Here's how the part is built. I have some questions about the finished solid (model axes, mm). A direction names the side the tool comes from. Round coordinates to 2 decimals unless told otherwise and drop trailing zeros. Write each loop counter-clockwise with the first axis right and the second up, starting at its lowest first coordinate (ties: lowest second). Pieces come first, ordered by that corner, then holes. Notation, with made-up numbers: M -13,-23 L 28,-23 A29 cw 28,16 Z; hole C 35,23 d5. An arc over 180 degrees is marked long. Use one line per item in the form item = value. Start each with the question number.
Q1. We'd pull the mould along X, two halves only. Please class faces 1 (the face through (-7, 12, 2)), 2 (the face through (-3.04, -11.29, -3.32)), 3 (the face through (-6.834, -8.007, -1.517)): +X half, -X half, draft (parallel to the pull), parting line (faces both ways), or undercut.
Q2. I need wall thicknesses on line 1 along X through (y, z) = (-11.4, 0); line 2 along Y through (x, z) = (-2.75, 6.5); line 3 along X through (y, z) = (6.5, 0). Which ranges of each line are inside material? Lowest first, please. Write a range as from..to.
Q3. I'm going to push flat-ended pins straight in: pin 1 Ø4.5 at (x, z) = (1.5, 2.5) entering from -Y; pin 2 Ø6 at (x, z) = (0.5, -2.5) entering from +Y; pin 3 Ø7 at (x, z) = (-3.5, 1) entering from +Y; pin 4 Ø1 at (x, y) = (4, -3.5) entering from -Z. Where does each tip first touch, or does it pass through?
Q4. For faces 4 (the face through (-3.905, 0.164, -0.867)), 5 (the face through (-7, -7.5, -2)), 6 (the face through (4.44, -10.9, -1.42)), 7 (the face through (-7, -12, 2)), 8 (the face through (6.64, 11.46, -1.47)), which set-ups out of +Z, -Z, +X, -X, +Y, -Y let a thin tool reach every point of the face, with its end or its side?
Q5. I want a section at C-C on z = 6.5. List the corners of the cut face in (x, y) for me, and give its area (3 significant figures).
Q6. I want a section at B-B on y = -10.25. List the corners of the cut face in (x, z) for me, and give its area (3 significant figures).
Q7. I want a section at A-A on z = -5.75. List the corners of the cut face in (x, y) for me, and give its area (3 significant figures).
```python
from build123d import *

# Parameters (mm, degrees)
SKETCH1_R           = 7.5
BOSS_EXTRUDE1_DEPTH = 12
SKETCH2_R           = 4
CUT_EXTRUDE1_DEPTH  = 24
CUT_EXTRUDE2_START  = -3.5
SKETCH3_R           = 7.5
SKETCH3_R_2         = 7
CUT_EXTRUDE2_DEPTH  = 1


with BuildPart() as part:
    # Sketch1 → Boss-Extrude1 (new, symmetric)
    with BuildSketch(Plane(origin=(0, 0, 0), x_dir=(1, 0, 0), z_dir=(0, 1, 0))):
        with Locations(Location((0, 0, 0), (0, 0, 270))):
            Circle(SKETCH1_R)
    extrude(amount=BOSS_EXTRUDE1_DEPTH, both=True)

    # Sketch2 → Cut-Extrude1 (cut)
    with BuildSketch(Plane(origin=(0, 12, 0), x_dir=(1, 0, 0), z_dir=(0, 1, 0))):
        with Locations(Location((0, 0, 0), (0, 0, 270))):
            Circle(SKETCH2_R)
    extrude(amount=-CUT_EXTRUDE1_DEPTH, mode=Mode.SUBTRACT)

    # Sketch3 → Cut-Extrude2 (cut)
    with BuildSketch(Plane(origin=(0, 12, 0), x_dir=(1, 0, 0), z_dir=(0, 1, 0)).offset(CUT_EXTRUDE2_START)):
        with Locations(Location((0, 0, 0), (0, 0, 270))):
            Circle(SKETCH3_R)
        with Locations(Location((0, 0, 0), (0, 0, 270))):
            Circle(SKETCH3_R_2, mode=Mode.SUBTRACT)
    cut_extrude2 = extrude(amount=-CUT_EXTRUDE2_DEPTH, mode=Mode.SUBTRACT)

    # Sketch4 → Cut-Revolve1 (revolve, cut)
    with BuildSketch(Plane(origin=(0, 0, 0), x_dir=(0, 0, -1), z_dir=(1, 0, 0)), mode=Mode.PRIVATE) as cut_revolve1_sk:
        Polygon((4, 12), (4, 11.7), (4.5, 11.7), (4.5, 10.9), (6.8, 10.9), (6.8, 12), align=None)
    cut_revolve1 = revolve(cut_revolve1_sk.sketch.rotate(Axis((0, 10.5, 0), (0, -1, 0)), 180), axis=Axis((0, 10.5, 0), (0, -1, 0)), mode=Mode.SUBTRACT)

    # Mirror1: Cut-Extrude2, Cut-Revolve1 across plane
    add(cut_extrude2.mirror(Plane.ZX), mode=Mode.SUBTRACT)
    add(cut_revolve1.mirror(Plane.ZX), mode=Mode.SUBTRACT)


solid = part.part
```
Reported:
q1.face_1 = draft
q1.face_2 = undercut
q1.face_3 = parting line
q2.line_1 = -7.5..-6.8, -4.5..-4, 4..4.5, 6.8..7.5
q2.line_2 = -12..-8.5, -7.5..7.5, 8.5..12
q2.line_3 = -7.5..-4, 4..7.5
q3.pin_1 = -11.7
q3.pin_2 = 11.7
q3.pin_3 = 12
q3.pin_4 = -6.63
q4.face_4 = +Y, -Y
q4.face_5 = none
q4.face_6 = -Y
q4.face_7 = +Z, -Z, +X, -X, -Y
q4.face_8 = +Y
q5.outline = M -3.74,-12 L -2,-12 L -2,-10.9 L 2,-10.9 L 2,-12 L 3.74,-12 L 3.74,-8.5 L 2.6,-8.5 L 2.6,-7.5 L 3.74,-7.5 L 3.74,7.5 L 2.6,7.5 L 2.6,8.5 L 3.74,8.5 L 3.74,12 L 2,12 L 2,10.9 L -2,10.9 L -2,12 L -3.74,12 L -3.74,8.5 L -2.6,8.5 L -2.6,7.5 L -3.74,7.5 L -3.74,-7.5 L -2.6,-7.5 L -2.6,-8.5 L -3.74,-8.5 Z
q5.area = 166 mm^2
q6.outline = C 0,0 d15; hole C 0,0 d8
q6.area = 126 mm^2
q7.outline = M -4.82,-12 L -3.63,-12 L -3.63,-10.9 L 3.63,-10.9 L 3.63,-12 L 4.82,-12 L 4.82,-8.5 L 3.99,-8.5 L 3.99,-7.5 L 4.82,-7.5 L 4.82,7.5 L 3.99,7.5 L 3.99,8.5 L 4.82,8.5 L 4.82,12 L 3.63,12 L 3.63,10.9 L -3.63,10.9 L -3.63,12 L -4.82,12 L -4.82,8.5 L -3.99,8.5 L -3.99,7.5 L -4.82,7.5 L -4.82,-7.5 L -3.99,-7.5 L -3.99,-8.5 L -4.82,-8.5 Z
q7.area = 212 mm^2
